Build history of the part. All positions in model axes, mm. A direction names the side the tool comes from. Round coordinates to 2 decimals unless told otherwise and drop trailing zeros. Write each loop counter-clockwise with the first axis right and the second up, starting at its lowest first coordinate (ties: lowest second). Pieces come first, ordered by that corner, then holes. Notation, with made-up numbers: M -7.75,4 L 40.25,4 A16 cw 40.25,15 Z; hole C -0.5,85.25 d8. An arc over 180 degrees is marked long. Write item = value, one per line. Start each with the question number.
Q1. Probe L1, parallel to X at y = 10.9, z = 0; L2, parallel to X at y = 14.05, z = 0; L3, parallel to X at y = 1, z = 12. List the from-to ranges inside material, lowest first.
Q2. Band-saw the part on C-C on y = 2.5. Write the cut outline in (x, z).
Q3. Drop flat-ended pins along their axis: P1, Ø6, axis at x = -10.5, y = 11, coming from the -Z side; P2, Ø1.8, axis at x = 0, z = 12.78, coming from the +Y side; P3, Ø6, axis at x = 0, z = 0.5, coming from the +Y side; P4, Ø5, axis at x = 7, y = 4, coming from the -Z side. Give the stop position or say it passes through.
Q4. Pull direction X, two halves, no side cores. Call faces 3 (the cylindrical face through (-2.685, 12.028, -0.596)), 4 (the flat face through (0, 0, 0)), 5 (the cylindrical face through (-5.554, 7.402, 13.394)): released by +X, released by -X, zero draft, split by the parting line, or undercut.
Q5. Band-saw the part on A-A on x = 0. State how many separate pieces and enclosed holes the cut face has, plus the area to 3 significant figures.
Q6. Tool access for faces 1 (the cylindrical face through (-0.488, 11.774, -0.108)), 2 (the flat face through (0, 15, 6)): list every direction of +Z, -Z, +X, -X, +Y, -Y with a clear straight run to the whole face (end or side of a thin tool).
```python
from build123d import *

# Parameters (mm, degrees)
SKETCH1_R           = 14.5
BOSS_EXTRUDE1_DEPTH = 15
SKETCH2_R           = 1.1
CUT_EXTRUDE1_DEPTH  = 15
CHAMFER1_SIZE       = 0.5
CHAMFER2_SIZE       = 0.5
SKETCH3_R           = 2.75
SKETCH3_R_2         = 0.5
CUT_EXTRUDE2_DEPTH  = 5
SKETCH4_R           = 4
CUT_EXTRUDE3_DEPTH  = 1
FILLET1_R           = 1
FILLET2_R           = 0.5


# Some blends are built 0.0001 mm under size
with BuildPart() as part:
    # Sketch1 → Boss-Extrude1 (new body)
    with BuildSketch(Plane(origin=(0, 0, 0), x_dir=(1, 0, 0), z_dir=(0, 1, 0))):
        with Locations(Location((0, 0, 0), (0, 0, 270))):
            Circle(SKETCH1_R)
    extrude(amount=BOSS_EXTRUDE1_DEPTH)

    # Sketch2 → Cut-Extrude1 (cut)
    with BuildSketch(Plane(origin=(0, 15, 0), x_dir=(1, 0, 0), z_dir=(0, 1, 0))):
        with Locations(Location((0, 12.781725236, 0), (0, 0, 270))):
            Circle(SKETCH2_R)
        with Locations(Location((0, -12.781725236, 0), (0, 0, 270))):
            Circle(SKETCH2_R)
    extrude(amount=-CUT_EXTRUDE1_DEPTH, mode=Mode.SUBTRACT)

    # Chamfer1
    chamfer1_edges = [part.edges().sort_by_distance(p)[0] for p in [
        (0, 15, -13.881725236),
        (0, 15, 11.681725236),
    ]]
    chamfer(chamfer1_edges, length=CHAMFER1_SIZE)

    # Chamfer2
    # the kernel refuses this chamfer: 0.5 mm, written as the material it takes off along each edge
    with BuildSketch(Plane(origin=(0, 0, 0), x_dir=(0, 0, 1), z_dir=(-1, 0, 0))) as chamfer2_piece_1:
        Polygon((14.5, CHAMFER2_SIZE), (14.5 - CHAMFER2_SIZE, 0), (14.5, 0), align=None)
    revolve(axis=Axis((0, 0, 0), (0, 1, 0)), mode=Mode.SUBTRACT)
    with BuildSketch(Plane(origin=(0, 15, 0), x_dir=(0, 0, 1), z_dir=(-1, 0, 0))) as chamfer2_piece_2:
        Polygon((14.5 - CHAMFER2_SIZE, 0), (14.5, -CHAMFER2_SIZE), (14.5, 0), align=None)
    revolve(axis=Axis((0, 15, 0), (0, 1, 0)), mode=Mode.SUBTRACT)

    # Sketch3 → Cut-Extrude2 (cut)
    with BuildSketch(Plane(origin=(0, 15, 0), x_dir=(1, 0, 0), z_dir=(0, 1, 0))):
        with Locations(Location((0, 0, 0), (0, 0, 270))):
            Circle(SKETCH3_R)
        with Locations(Location((0, 0, 0), (0, 0, 270))):
            Circle(SKETCH3_R_2, mode=Mode.SUBTRACT)
    extrude(amount=-CUT_EXTRUDE2_DEPTH, mode=Mode.SUBTRACT)

    # Sketch4 → Cut-Extrude3 (cut)
    with BuildSketch(Plane(origin=(0, 15, 0), x_dir=(1, 0, 0), z_dir=(0, 1, 0))):
        with Locations(Location((0, 0, 0), (0, 0, 270))):
            Circle(SKETCH4_R)
    extrude(amount=-CUT_EXTRUDE3_DEPTH, mode=Mode.SUBTRACT)

    # Fillet1
    fillet1_edges = [part.edges().sort_by_distance(p)[0] for p in [
        (0, 15, -4),
    ]]
    fillet(fillet1_edges, radius=FILLET1_R - 0.0001)  # a hair under: the kernel refuses the full size

    # Fillet2
    fillet2_edges = [part.edges().sort_by_distance(p)[0] for p in [
        (0, 14, -0.5),
    ]]
    fillet(fillet2_edges, radius=FILLET2_R)


solid = part.part
```
Conclusion:
q1.L1 = -14.5 to -2.75, -0.5 to 0.5, 2.75 to 14.5
q1.L2 = -14.5 to -4, 4 to 14.5
q1.L3 = -8.14 to -0.77, 0.77 to 8.14
q2.outline = C 0,0 d29; hole C 0,-12.78 d2.2; hole C 0,12.78 d2.2
q3.P1 = -12.41
q3.P2 = through
q3.P3 = 14
q3.P4 = -13.78
q4.face_3 = undercut
q4.face_4 = zero draft
q4.face_5 = split by the parting line
q5.separate_pieces = 3
q5.enclosed_holes = 0
q5.area = 342 mm^2
q6.face_1 = +Y
q6.face_2 = +Z, -Z, +X, -X, +Y
